```python
from build123d import *

# Parameters (mm, degrees)
F0_W     = 50
F0_H     = 45
F1_DEPTH = 25
F3_DEPTH = 12
F4_R     = 5


with BuildPart() as f1:
    # F0 (on Top) → F1 (new body)
    with BuildSketch(Plane.XY):
        with Locations((2.5, 2.5)):
            Rectangle(F0_W, F0_H)
    extrude(amount=F1_DEPTH)

    # F2 (on face) → F3 (cut)
    with BuildSketch(Plane.XY.offset(25)):
        with BuildLine():
            ThreePointArc((1.5188633246, -4.0508734179), (1.5351749633, -3.8134761459), (1.5406159691, -3.5755813587))
            ThreePointArc((1.5406159691, -3.5755813587), (1.2521629282, -1.8671692612), (0.4187848362, -0.3481702463))
            ThreePointArc((0.4187848362, -0.3481702463), (0.7408484381, -2.2672537264), (1.5188633246, -4.0508734179))
        make_face()
        with BuildLine():
            ThreePointArc((0.4187848362, -0.3481702463), (1.2521629282, -1.8671692612), (1.5406159691, -3.5755813587))
            ThreePointArc((1.5406159691, -3.5755813587), (1.5351749633, -3.8134761459), (1.5188633246, -4.0508734179))
            ThreePointArc((1.5188633246, -4.0508734179), (10.4718881616, -7.6790094348), (16.3330176423, 0))
            ThreePointArc((16.3330176423, 0), (12.8314237876, 6.5947473606), (5.4069776088, 7.3881269744))
            Line((5.4069776088, 7.3881269744), (5.4069776088, 1.5949606824))
            Line((5.4069776088, 1.5949606824), (0.5725780424, 1.5949606824))
            ThreePointArc((0.5725780424, 1.5949606824), (0.4359857319, 0.628119961), (0.4187848362, -0.3481702463))
        make_face()
        with BuildLine():
            ThreePointArc((1.5188633246, -4.0508734179), (0.7408484381, -2.2672537264), (0.4187848362, -0.3481702463))
            ThreePointArc((0.4187848362, -0.3481702463), (-1.1358159194, 0.9730272564), (-3.078892131, 1.5949606824))
            ThreePointArc((-3.078892131, 1.5949606824), (-7.6975474715, -6.8613357478), (1.5188633246, -4.0508734179))
        make_face()
        with BuildLine():
            ThreePointArc((-3.078892131, 1.5949606824), (-1.1358159194, 0.9730272564), (0.4187848362, -0.3481702463))
            ThreePointArc((0.4187848362, -0.3481702463), (0.4359857319, 0.628119961), (0.5725780424, 1.5949606824))
            Line((0.5725780424, 1.5949606824), (-3.078892131, 1.5949606824))
        make_face()
        with BuildLine():
            Line((-3.078892131, 18.0523265153), (-3.078892131, 1.5949606824))
            Line((-3.078892131, 1.5949606824), (0.5725780424, 1.5949606824))
            ThreePointArc((0.5725780424, 1.5949606824), (2.2598502763, 5.1006686576), (5.4069776088, 7.3881269744))
            Line((5.4069776088, 7.3881269744), (5.4069776088, 18.0523265153))
            Line((5.4069776088, 18.0523265153), (-3.078892131, 18.0523265153))
        make_face()
        with BuildLine():
            ThreePointArc((5.4069776088, 7.3881269744), (2.2598502763, 5.1006686576), (0.5725780424, 1.5949606824))
            Line((0.5725780424, 1.5949606824), (5.4069776088, 1.5949606824))
            Line((5.4069776088, 1.5949606824), (5.4069776088, 7.3881269744))
        make_face()
    extrude(amount=-F3_DEPTH, mode=Mode.SUBTRACT)

    # F4
    f4_edges = [f1.edges().sort_by_distance(p)[0] for p in [
        (-22.5, 2.5, 0),
        (2.5, 25, 0),
        (2.5, -20, 0),
        (27.5, 2.5, 0),
    ]]
    fillet(f4_edges, radius=F4_R)


solid = f1.part
```
Geometry: final body of the model. Coordinates: model frame, mm. A direction names the side the tool comes from. Round coordinates to 2 decimals unless told otherwise and drop trailing zeros. Loops run counter-clockwise (first coordinate to the right, second up) from the corner with the lowest first, then second, coordinate; pieces in that order, holes last. Notation, with made-up numbers: (-31, 58.25) -> (-24, 58.25) arc R19 cw to (-24, 63.25) -> close; hole circle Ø9 at (22, -8.75). An arc over 180 degrees is marked (long way). Use one line per item in the form item = value.
Item 1: Contact query for a flat-ended pin moving along its axis: pin 1 Ø9.5 at (x, y) = (-3.66, -3.58) entering from +Z. Output: stop coordinate, or through.
Evaluation:
pin_1 = 13
Item 2: Cut plane D-D on y = -7. Output: boundary loops of the cut face in (x, z).
Evaluation:
outline = (-22.5, 5) arc R5 ccw to (-17.5, 0) -> (22.5, 0) arc R5 ccw to (27.5, 5) -> (27.5, 25) -> (12.16, 25) -> (12.16, 13) -> (4.58, 13) -> (4.58, 25) -> (0.25, 25) -> (0.25, 13) -> (-7.58, 13) -> (-7.58, 25) -> (-22.5, 25) -> close
Item 3: Material intervals for probe 1 along Y at (x, z) = (8, 14.25); probe 2 along Z at (x, y) = (-2.5, 16); probe 3 along X at (y, z) = (7, 17), sorted ascending.
Evaluation:
probe_1 = -20 to -7.95, 7.95 to 25
probe_2 = 0 to 13
probe_3 = -22.5 to -3.08, 12.16 to 27.5
Item 4: Access query for faces 1 (the flat face through (2, 3, 0)), 2 (the flat face through (-3.079, 10, 19)). Directions: +Z, -Z, +X, -X, +Y, -Y. A direction counts if a zero-diameter tool reaches every point of the face in a straight line with its end or side. Return the directions, or none.
Evaluation:
face_1 = -Z, +X, -X, +Y, -Y
face_2 = +Z
Item 5: Draft query along X for faces 3 (the cylindrical face through (3, -19, 2)), 4 (the cylindrical face through (26, 2.82, 1.43)), 5 (the flat face through (4, 2, 13)), 6 (the flat face through (-22.5, 2, 15)). Return one class per face: released by +X, released by -X, zero draft, split by the parting line, or undercut.
Evaluation:
face_3 = zero draft
face_4 = released by +X
face_5 = undercut
face_6 = released by -X
Item 6: Cut plane C-C on x = 15.5. Output: boundary loops of the cut face in (y, z), then the cut area to 3 significant figures.
Evaluation:
outline = (-20, 5) arc R5 ccw to (-15, 0) -> (20, 0) arc R5 ccw to (25, 5) -> (25, 25) -> (3.55, 25) -> (3.55, 13) -> (-3.55, 13) -> (-3.55, 25) -> (-20, 25) -> close
area = 1,030 mm2
Item 7: Cut plane A-A on z = 14.5. Output: boundary loops of the cut face in (x, y), then the cut area to 3 significant figures.
Evaluation:
outline = (-22.5, -20) -> (27.5, -20) -> (27.5, 25) -> (-22.5, 25) -> close; hole (-3.08, 1.59) arc R5.2 ccw (long way) to (1.52, -4.05) arc R7.96 ccw (long way) to (5.41, 7.39) -> (5.41, 18.05) -> (-3.08, 18.05) -> close
area = 1,840 mm2
Item 8: Cut plane B-B on y = 12. Output: boundary loops of the cut face in (x, z), then the cut area to 3 significant figures.
Evaluation:
outline = (-22.5, 5) arc R5 ccw to (-17.5, 0) -> (22.5, 0) arc R5 ccw to (27.5, 5) -> (27.5, 25) -> (5.41, 25) -> (5.41, 13) -> (-3.08, 13) -> (-3.08, 25) -> (-22.5, 25) -> close
area = 1,140 mm2
